```python
from build123d import *

# Parameters (mm, degrees)
CROQUIS2_R              = 35
SALIENTE_EXTRUIR1_DEPTH = 3


with BuildPart() as part:
    # Croquis2 → Saliente-Extruir1 (new body)
    with BuildSketch(Plane.XY):
        with BuildLine():
            Line((-65, 0), (-32.5, -56.291651246))
            Line((-32.5, -56.291651246), (32.5, -56.291651246))
            Line((32.5, -56.291651246), (65, 0))
            Line((65, 0), (32.5, 56.291651246))
            Line((32.5, 56.291651246), (-32.5, 56.291651246))
            ThreePointArc((-32.5, 56.291651246), (-31.127404736, 51.169055982), (-36.25, 49.796460718))
            Line((-36.25, 49.796460718), (-65, 0))
        make_face()
        Circle(CROQUIS2_R, mode=Mode.SUBTRACT)
    extrude(amount=SALIENTE_EXTRUIR1_DEPTH)


solid = part.part
```
Source: CAD feature listing. Evaluate the final solid. Frame: model axes, mm. Give positions to 0.01 mm unless a question says otherwise; leave off trailing zeros. Loops run counter-clockwise (first coordinate to the right, second up) from the corner with the lowest first, then second, coordinate; pieces in that order, holes last. Notation, with made-up numbers: (-6, -22) - (53, -22) arc R15 ccw to (53, -18) - close; hole circle Ø7 at (65.5, -18). An arc over 180 degrees is marked (long way). Use CSV: the item, a comma, the result in double quotes.
1) Mould query, pull axis X, two halves, no side actions, for faces 1 (the flat face through (48.522, -28.54, 1.479)), 2 (the flat face through (0, -56.292, 1)), 3 (the flat face through (-50.42, 25.25, 1.48)), 4 (the cylindrical face through (-31.087, 51.241, 1.479)). Classes: +X half, -X half, draft (parallel to the pull), parting line (faces both ways), or undercut.
Worked out:
face 1,"+X half"
face 2,"draft"
face 3,"-X half"
face 4,"undercut"
2) Cut plane D-D (y = 36.5). Output: boundary loops of the cut face in (x, z), and give its area (3 significant figures).
Worked out:
outline,"(-43.93, 0) - (43.93, 0) - (43.93, 3) - (-43.93, 3) - close"
area,"264 mm^2"
3) Cut plane C-C (z = 1.45). Output: boundary loops of the cut face in (x, y) (3 decimals).
Worked out:
outline,"(-65, 0) - (-32.5, -56.292) - (32.5, -56.292) - (65, 0) - (32.5, 56.292) - (-32.5, 56.292) arc R3.75 cw to (-36.25, 49.796) - close; hole circle Ø70 at (0, 0)"
4) Line query: line 1 (Y direction, x = 0, z = 1.1); line 2 (Y direction, x = 11, z = 1); line 3 (X direction, y = -9, z = 1.65). Output: solid intervals per line, ascending.
Worked out:
line 1,"y = -56.29 to -35, 35 to 56.29"
line 2,"y = -56.29 to -33.23, 33.23 to 56.29"
line 3,"x = -59.8 to -33.82, 33.82 to 59.8"
5) Pin query (flat end, axial travel): P1, Ø1.5, axis at x = 34, z = 1.5, coming from the -Y side; P2, Ø1.5, axis at y = 10.5, z = 1, coming from the +X side; P3, Ø1, axis at y = 32.5, z = 2.5, coming from the -X side. Return the tip coordinate at first contact, or that it passes through.
Worked out:
P1,"stops at y = -54.99"
P2,"stops at x = 59.37"
P3,"stops at x = -46.52"
6) Cut plane A-A (x = -21). Output: boundary loops of the cut face in (y, z).
Worked out:
outline,"(-56.29, 0) - (-28, 0) - (-28, 3) - (-56.29, 3) - close; (28, 0) - (56.29, 0) - (56.29, 3) - (28, 3) - close"
7) Cut plane B-B (y = -29). Output: boundary loops of the cut face in (x, z).
Worked out:
outline,"(-48.26, 0) - (-19.6, 0) - (-19.6, 3) - (-48.26, 3) - close; (19.6, 0) - (48.26, 0) - (48.26, 3) - (19.6, 3) - close"
